Build history of the part. All positions in model axes, mm. A direction names the side the tool comes from. Round coordinates to 2 decimals unless told otherwise and drop trailing zeros. Loops run counter-clockwise (first coordinate to the right, second up) from the corner with the lowest first, then second, coordinate; pieces in that order, holes last. Notation, with made-up numbers: M 31.25,-14.5 L 40.25,-14.5 A31 ccw 40.25,18.5 Z; hole C 14,-38.75 d10. An arc over 180 degrees is marked long. One line per item, written item: value.
```python
from build123d import *

# Parameters (mm, degrees)
CROQUIS1_W                                           = 43
CROQUIS1_H                                           = 39
SALIENTE_EXTRUIR1_DEPTH                              = 2.5
AVELLANADO_PARA_TORNILLO_CON_CABEZA_AVEL_D           = 3.4
AVELLANADO_PARA_TORNILLO_CON_CABEZA_AVEL_DEPTH       = 12
AVELLANADO_PARA_TORNILLO_CON_CABEZA_AVEL_CSINK_D     = 6.94
AVELLANADO_PARA_TORNILLO_CON_CABEZA_AVEL_CSINK_ANGLE = 90
AVELLANADO_PARA_TORNILLO_CON_CABEZA_AVEL_TIP         = 1.021463052
CROQUIS6_W                                           = 5
CROQUIS6_H                                           = 1
SALIENTE_EXTRUIR2_DEPTH                              = 1.5
REDONDEO1_R                                          = 0.6


with BuildPart() as part:
    # Croquis1 → Saliente-Extruir1 (new body)
    with BuildSketch(Plane.XY):
        Rectangle(CROQUIS1_W, CROQUIS1_H)
    extrude(amount=SALIENTE_EXTRUIR1_DEPTH)

    # Avellanado para tornillo con cabeza avellanada de clavija hexagonal de M31
    with Locations(Plane(origin=(-15.5, 14.5, 2.5), x_dir=(1, 0, 0), z_dir=(0, 0, 1))):
        with Locations((0, 0), (31, 0)):
            CounterSinkHole(AVELLANADO_PARA_TORNILLO_CON_CABEZA_AVEL_D / 2, AVELLANADO_PARA_TORNILLO_CON_CABEZA_AVEL_CSINK_D / 2, depth=AVELLANADO_PARA_TORNILLO_CON_CABEZA_AVEL_DEPTH, counter_sink_angle=AVELLANADO_PARA_TORNILLO_CON_CABEZA_AVEL_CSINK_ANGLE)
            with Locations((0, 0, -(AVELLANADO_PARA_TORNILLO_CON_CABEZA_AVEL_DEPTH + AVELLANADO_PARA_TORNILLO_CON_CABEZA_AVEL_TIP / 2))):  # 118° drill point
                Cone(0, AVELLANADO_PARA_TORNILLO_CON_CABEZA_AVEL_D / 2, AVELLANADO_PARA_TORNILLO_CON_CABEZA_AVEL_TIP, mode=Mode.SUBTRACT)

    # Croquis6 → Saliente-Extruir2 (add)
    with BuildSketch(Plane.XZ.offset(19.5)):
        with Locations((-16.5, 1.25)):
            Rectangle(CROQUIS6_W, CROQUIS6_H)
        with Locations((16.5, 1.25)):
            Rectangle(CROQUIS6_W, CROQUIS6_H)
    extrude(amount=SALIENTE_EXTRUIR2_DEPTH)

    # Redondeo1
    redondeo1_edges = [part.edges().sort_by_distance(p)[0] for p in [
        (21.5, -19.5, 1.25),
        (-21.5, -19.5, 1.25),
        (-21.5, 19.5, 1.25),
        (21.5, 19.5, 1.25),
    ]]
    fillet(redondeo1_edges, radius=REDONDEO1_R)


solid = part.part
```
Item 1: Slice it at A-A, the plane x = 15.5. Give the cut face in (y, z).
Check values:
outline: M -21,0.75 L -19.5,0.75 L -19.5,0 L 12.8,0 L 12.8,0.73 L 11.03,2.5 L -19.5,2.5 L -19.5,1.75 L -21,1.75 Z; M 16.2,0 L 19.5,0 L 19.5,2.5 L 17.97,2.5 L 16.2,0.73 Z
Item 2: Slice it at C-C, the plane x = 1.5. Give the cut face in (y, z), and give its area (3 significant figures).
Check values:
outline: M -19.5,0 L 19.5,0 L 19.5,2.5 L -19.5,2.5 Z
area: 97.5 mm2
Item 3: Slice it at B-B, the plane y = 14.5. Give the cut face in (x, z), and give its area (3 significant figures).
Check values:
outline: M -21.5,0 L -17.2,0 L -17.2,0.73 L -18.97,2.5 L -21.5,2.5 Z; M -13.8,0 L 13.8,0 L 13.8,0.73 L 12.03,2.5 L -12.03,2.5 L -13.8,0.73 Z; M 17.2,0 L 21.5,0 L 21.5,2.5 L 18.97,2.5 L 17.2,0.73 Z
area: 84.2 mm2
Item 4: Drop flat-ended pins along their axis: P1, Ø4, axis at x = 15.5, y = 14.5, coming from the +Z side; P2, Ø3, axis at x = -16, y = 11, coming from the -Z side; P3, Ø0.8, axis at y = -20, z = 1, coming from the +X side; P4, Ø1.2, axis at x = 17, y = -20.5, coming from the +Z side. Give the stop position or say it passes through.
Check values:
P1: stops at z = 1.03
P2: stops at z = 0
P3: stops at x = 19
P4: stops at z = 1.75
Item 5: Pull direction Y, two halves, no side cores. Call faces 1 (the face through (16, -21, 1)), 2 (the face through (0, 0, 2.5)), 3 (the face through (0, 19.5, 1)), 4 (the face through (-17.07, 13.85, 0.36)): pulls with the +Y half, pulls with the -Y half, needs draft (parallel to the pull), parting line crosses it, or undercut.
Check values:
face 1: pulls with the -Y half
face 2: needs draft
face 3: pulls with the +Y half
face 4: undercut
Item 6: Wall check: line 1 along X through (y, z) = (14.5, 0.25); line 2 along Y through (x, z) = (-15.5, 0.25); line 3 along X through (y, z) = (16, 0.8). Give the ranges that are in metal, low to high.
Check values:
line 1: x = -21.5 to -17.2, -13.8 to 13.8, 17.2 to 21.5
line 2: y = -19.5 to 12.8, 16.2 to 19.5
line 3: x = -21.5 to -16.44, -14.56 to 14.56, 16.44 to 21.5
Item 7: Which spindle directions (+Z, -Z, +X, -X, +Y, -Y) get a long thin tool onto all of the face, cutting with end or side? Do faces 5 (the face through (16, -20, 1.75)), 6 (the face through (16, -20, 0.75)), 7 (the face through (14, -20, 1)). Say none if no direction does.
Check values:
face 5: +Z, +X, -X, -Y
face 6: -Z, +X, -X, -Y
face 7: +Z, -Z, -Y
